Can you work these out from the model? Positions are in its coordinate system, mm. A direction names the side the tool comes from. Round coordinates to 2 decimals unless told otherwise and drop trailing zeros. Loops run counter-clockwise (first coordinate to the right, second up) from the corner with the lowest first, then second, coordinate; pieces in that order, holes last.
Autodesk Inventor part; units mm, degrees
ref_plane "YZ Plane" through (0, 0, 0) normal (1, 0, 0) x (0, 1, 0)
ref_plane "XZ Plane" through (0, 0, 0) normal (0, 1, 0) x (-1, 0, 0)
ref_plane "XY Plane" through (0, 0, 0) normal (0, 0, 1) x (1, 0, 0)
sketch "Sketch1" plane through (0, 0, 0) normal (0, 1, 0) x (-1, 0, 0)
  line L0 (21.3, 34.3) -> (-21.3, 34.3)
  line L1 (-21.3, 34.3) -> (-21.3, -34.3)
  line L2 (-21.3, -34.3) -> (21.3, -34.3)
  line L3 (21.3, -34.3) -> (21.3, 34.3)
  line L4 (21.3, 34.3) -> (-21.3, -34.3) construction
  line L5 (-21.3, 34.3) -> (21.3, -34.3) construction
  point P0 (0, 0)
  dimension "d0" = 42.6
  dimension "d1" = 68.6
extrude "Extrusion1" add sketch "Sketch1" along normal blind 7
sketch "Sketch2" plane through (0, 7, 0) normal (0, 1, 0) x (1, 0, 0)
  line L0 (-19.75, -32.75) -> (19.75, -32.75)
  line L1 (19.75, -32.75) -> (19.75, 32.75)
  line L2 (19.75, 32.75) -> (-19.75, 32.75)
  line L3 (-19.75, 32.75) -> (-19.75, -32.75)
  line L4 (-19.75, -32.75) -> (19.75, 32.75) construction
  line L5 (19.75, -32.75) -> (-19.75, 32.75) construction
  point P0 (0, 0)
  dimension "d4" = 39.5
  dimension "d5" = 65.5
extrude "Extrusion2" cut sketch "Sketch2" against normal blind 1.6
sketch "Sketch3" plane through (0, 5.4, 0) normal (0, 1, 0) x (1, 0, 0)
  line L0 (-18.05, -31.05) -> (18.05, -31.05)
  line L1 (18.05, -31.05) -> (18.05, 31.05)
  line L2 (18.05, 31.05) -> (-18.05, 31.05)
  line L3 (-18.05, 31.05) -> (-18.05, -31.05)
  line L4 (-18.05, -31.05) -> (18.05, 31.05) construction
  line L5 (18.05, -31.05) -> (-18.05, 31.05) construction
  point P0 (0, 0)
  dimension "d8" = 36.1
  dimension "d9" = 62.1
extrude "Extrusion3" cut sketch "Sketch3" against normal blind 3.4
sketch "Sketch4" plane through (0, 2, 0) normal (0, 1, 0) x (1, 0, 0)
  circle A0 centre (-15.6, 28.6) radius 4
  circle A1 centre (15.6, 28.6) radius 4
  circle A2 centre (-15.6, -28.6) radius 4
  circle A3 centre (15.6, -28.6) radius 4
  line L0 (-18.05, 31.05) -> (18.05, 31.05)
  line L1 (-18.05, -31.05) -> (-18.05, 31.05)
  point P0 (0, 0)
  dimension "d12" = 31.2
  dimension "d13" = 31.2
  dimension "d14" = 57.2
  dimension "d15" = 57.2
  dimension "d16" = 8
  dimension "d17" = 8
  dimension "d18" = 8
  dimension "d19" = 8
  dimension "d22" = 0
  dimension "d23" = 15.6
  dimension "d24" = 28.6
  dimension "d25" = 0
extrude "Extrusion4" add sketch "Sketch4" along normal blind 3.4
sketch "Sketch5" plane through (-15.6, 5.4, -28.6) normal (0, 1, 0) x (0.7071068, 0, -0.7071068)
  arc A0 (-3.9682, -0.5034) -> (3.9682, -0.5034) centre (0, 0) ccw
  circle A1 centre (0, 0) radius 1
  arc A2 (21.5584, -18.0935) -> (21.5584, -26.0299) centre (22.0617, -22.0617) ccw
  circle A3 centre (22.0617, -22.0617) radius 1
  arc A4 (-14.4166, -62.0049) -> (-22.353, -62.0049) centre (-18.3848, -62.5082) ccw
  circle A5 centre (-18.3848, -62.5082) radius 1
  arc A6 (-39.9431, -44.4147) -> (-39.9431, -36.4783) centre (-40.4465, -40.4465) ccw
  circle A7 centre (-40.4465, -40.4465) radius 1
  point P0 (-9.1924, -31.2541)
  point P1 (-0.6856, -2.9206)
  point P2 (0.6856, -2.9206)
  point P3 (-24.8409, 22.606)
  point P4 (-24.8409, 21.2347)
  point P5 (19.0704, 65.146)
  point P6 (17.6991, 65.146)
  dimension "d28" = 2
  dimension "d29" = 2
  dimension "d30" = 2
  dimension "d31" = 2
extrude "Extrusion5" cut sketch "Sketch5" against normal blind 3.6
fillet "Fillet3" radius 2 8 edges at (-19.75, 6.2, -32.75) (19.75, 6.2, -32.75) (-19.75, 6.2, 32.75) (19.75, 6.2, 32.75) (-21.3, 3.5, -34.3) (-21.3, 3.5, 34.3) (21.3, 3.5, 34.3) (21.3, 3.5, -34.3)
sketch "Sketch8" plane through (21.3, 0, 32.3) normal (1, 0, 0) x (0, 0, -1)
  line L0 (63.05, 7) -> (1.55, 7)
  line L1 (0, 0) -> (64.6, 0)
  line L2 (39.8, 7) -> (24.8, 7)
  line L3 (24.8, 7) -> (24.8, 0)
  line L4 (24.8, 0) -> (39.8, 0)
  line L5 (39.8, 0) -> (39.8, 7)
  point P0 (32.3, 0)
  point P1 (39.8, 0)
  point P2 (24.8, 7)
  dimension "d49" = 15
  dimension "d50" = 7.5
extrude "Extrusion7" add sketch "Sketch8" along normal blind 15
sketch "Sketch9" plane through (0, 7, 0) normal (0, 1, 0) x (1, 0, 0)
  line L0 (36.3, 7.5) -> (36.3, -7.5)
  point P0 (0, 0)
  point P1 (28.8, 0.0728)
  dimension "d60" = 7.5
hole "Hole2" at (28.8, 7, -0.0728) direction (0, -1, 0) diameter 6.756 end through all counterbore diameter 11.113 counterbore depth 6.35
fillet "Fillet4" radius 3.5 2 edges at (21.3, 3.5, -7.5) (21.3, 3.5, 7.5)
fillet "Fillet5" radius 7.5 2 edges at (36.3, 3.5, 7.5) (36.3, 3.5, -7.5)
equation "\"d13\" = d12"
equation "\"d14\" = d15"
properties part number "Thermister_Amp_Mount"
(1) Will these pins go through, and if not, where does the flat tip stop? P1, Ø1, axis at x = 4, z = 4.5, coming from the -Y side; P2, Ø2, axis at y = 3, z = -17.5, coming from the +X side; P3, Ø2, axis at x = -15.5, z = -29, coming from the +Y side; P4, Ø3, axis at x = 26.5, y = 2, coming from the +Z side.
Worked answers:
P1: stops at y = 0
P2: stops at x = 21.3
P3: stops at y = 5.4
P4: stops at z = 7.5
(2) If I drill on line 1 (Z direction, x = -15.6, y = 4.75); line 2 (X direction, y = 4.35, z = -28.6); line 3 (Z direction, x = -6.5, y = 6), over which ranges is the centre line in solid material (lowest first)?
Worked answers:
line 1: z = -34.3 to -29.6, -27.6 to -24.6, 24.6 to 27.6, 29.6 to 34.3
line 2: x = -21.3 to -16.6, -14.6 to -11.6, 11.6 to 14.6, 16.6 to 21.3
line 3: z = -34.3 to -32.75, 32.75 to 34.3
(3) If we mould it in two halves opening along Z, with no side actions, what happens to faces 1 (the flat face through (20, 7, 0)), 2 (the flat face through (32.4, 0.65, -0.2)), 3 (the cylindrical face through (34.161, 3.451, 5.245))? For each: released by +Z, released by -Z, zero draft, split by the parting line, or undercut.
Worked answers:
face 1: zero draft
face 2: undercut
face 3: released by +Z
(4) If we section it at A-A, the plane x = 30: List the corners of the cut face in (y, z) for me, then the cut area to 3 significant figures.
Worked answers:
outline: (0, -7.4) - (7, -7.4) - (7, -5.5) - (0.65, -5.5) - (0.65, -3.23) - (0, -3.23) - close; (0, 3.08) - (0.65, 3.08) - (0.65, 5.35) - (7, 5.35) - (7, 7.4) - (0, 7.4) - close
area: 30.6 mm2
(5) If we section it at C-C, the plane x = -3.5: List the corners of the cut face in (y, z) for me.
Worked answers:
outline: (0, -34.3) - (7, -34.3) - (7, -32.75) - (5.4, -32.75) - (5.4, -31.05) - (2, -31.05) - (2, 31.05) - (5.4, 31.05) - (5.4, 32.75) - (7, 32.75) - (7, 34.3) - (0, 34.3) - close
(6) If we section it at B-B, the plane z = 21: List the corners of the cut face in (x, y) for me.
Worked answers:
outline: (-21.3, 0) - (21.3, 0) - (21.3, 7) - (19.75, 7) - (19.75, 5.4) - (18.05, 5.4) - (18.05, 2) - (-18.05, 2) - (-18.05, 5.4) - (-19.75, 5.4) - (-19.75, 7) - (-21.3, 7) - close
(7) For faces 4 (the flat face through (0, 2, 0)), 5 (the flat face through (21.3, 3, -22)), 6 (the flat face through (21.3, 3, 22)), which set-ups out of +Z, -Z, +X, -X, +Y, -Y let a thin tool reach every point of the face, with its end or its side?
Worked answers:
face 4: +Y
face 5: -Z, +X, +Y, -Y
face 6: +Z, +X, +Y, -Y
(8) If we section it at D-D, the plane y = 3.75: State how many separate pieces and enclosed holes the cut face has, then the cut area to 3 significant figures.
Worked answers:
separate pieces: 1
enclosed holes: 6
area: 921 mm2
